Verification items for the finished model (mm, model axes). A direction names the side the tool comes from. Round coordinates to 2 decimals unless told otherwise and drop trailing zeros. Loops run counter-clockwise (first coordinate to the right, second up) from the corner with the lowest first, then second, coordinate; pieces in that order, holes last. Notation, with made-up numbers: (23.5, 30.5) -> (76.5, 30.5) arc R16 cw to (76.5, 43.5) -> close; hole circle Ø4 at (9, -32.5). An arc over 180 degrees is marked (long way). Write item = value, one per line.
Autodesk Inventor part; units mm, degrees
ref_plane "YZ Plane" through (0, 0, 0) normal (1, 0, 0) x (0, 1, 0)
ref_plane "XZ Plane" through (0, 0, 0) normal (0, 1, 0) x (-1, 0, 0)
ref_plane "XY Plane" through (0, 0, 0) normal (0, 0, 1) x (1, 0, 0)
sketch "Sketch1" plane through (0, 0, 0) normal (0, 1, 0) x (-1, 0, 0)
  circle A0 centre (0, 0) radius 9.5
  dimension "d0" = 19
extrude "Extrusion1" add sketch "Sketch1" along normal blind 1.4
sketch "Sketch2" plane through (0, 1.4, 0) normal (0, 1, 0) x (1, 0, 0)
  circle A0 centre (0, 0) radius 9.5
  circle A1 centre (0, 0) radius 3.6
  dimension "d3" = 7.2
extrude "Extrusion2" add sketch "Sketch2" along normal blind 42 contours A1
sketch "Sketch3" plane through (0, 43.4, 0) normal (0, 1, 0) x (1, 0, 0)
  circle A0 centre (0, 0) radius 3.6
  line L0 (-3.1177, -1.8) -> (3.1177, -1.8)
  arc A1 (-3.1177, -1.8) -> (3.1177, -1.8) centre (0, 0) ccw
  dimension "d6" = 1.8
extrude "Extrusion3" cut sketch "Sketch3" against normal blind 14.4 contours L0 A0 picked at (0.1393, -2.8389)
sketch "Sketch4" plane through (-3.1177, 43.4, 1.8) normal (0, 0, 1) x (1, 0, 0)
  line L0 (0, 0) -> (6.2354, 0)
  circle A0 centre (3.1177, -3.2) radius 1.2
  point P0 (3.1177, -43.4)
  dimension "d9" = 2.4
  dimension "d10" = 3.2
extrude "Extrusion4" cut sketch "Sketch4" against normal through all
properties part number "Front Axle"
(1) Sectioned sample at B-B, the plane z = 0. Record the cut outline in (x, y).
Filled sheet:
outline = (-9.5, 0) -> (9.5, 0) -> (9.5, 1.4) -> (3.6, 1.4) -> (3.6, 43.4) -> (-3.6, 43.4) -> (-3.6, 1.4) -> (-9.5, 1.4) -> close; hole circle Ø2.4 at (0, 40.2)
(2) Sectioned sample at A-A, the plane x = 0. Record the cut outline in (y, z), and give its area (3 significant figures).
Filled sheet:
outline = (0, -9.5) -> (1.4, -9.5) -> (1.4, -3.6) -> (39, -3.6) -> (39, 1.8) -> (29, 1.8) -> (29, 3.6) -> (1.4, 3.6) -> (1.4, 9.5) -> (0, 9.5) -> close; (41.4, -3.6) -> (43.4, -3.6) -> (43.4, 1.8) -> (41.4, 1.8) -> close
area = 290 mm2
(3) Go/stop test with flat-tipped pins: pin 1 Ø2 at (x, z) = (-0.5, 3) entering from +Y; pin 2 Ø1 at (x, y) = (5.5, 26.5) entering from -Z; pin 3 Ø10 at (x, y) = (-4.5, 8) entering from -Z; pin 4 Ø3 at (x, y) = (0, 40.2) entering from +Z. Record where each tip stops, or that it passes through.
Filled sheet:
pin_1 = 29
pin_2 = through
pin_3 = -3.6
pin_4 = 1.8
(4) Material ranges on probe 1 along Y at (x, z) = (0, 0.25); probe 2 along X at (y, z) = (40.2, -0.1); probe 3 along Y at (x, z) = (-1, 3.75), recorded low to high. Write a range as from..to.
Filled sheet:
probe_1 = 0..39, 41.4..43.4
probe_2 = -3.6..-1.2, 1.2..3.6
probe_3 = 0..1.4
(5) Sectioned sample at C-C, the plane y = 40.2. Record the cut outline in (x, z), and give its area (3 significant figures).
Filled sheet:
outline = (-3.12, 1.8) arc R3.6 ccw to (-1.2, -3.39) -> (-1.2, 1.8) -> close; (1.2, -3.39) arc R3.6 ccw to (3.12, 1.8) -> (1.2, 1.8) -> close
area = 20.0 mm2
(6) Sectioned sample at D-D, the plane y = 21.5. Record the cut outline in (x, z).
Filled sheet:
outline = circle Ø7.2 at (0, 0)
(7) Set-up check for faces 1 (the face through (-4.38, 0.69, 8.43)), 2 (the face through (0, 29, 2)), 3 (the face through (0, 1.4, -4)): record each of +Z, -Z, +X, -X, +Y, -Y from which the full face is reachable in a straight line by a thin tool's end or side.
Filled sheet:
face_1 = +Y, -Y
face_2 = +Z, +X, -X, +Y
face_3 = +Y
